Build history of the part. All positions in model axes, mm. A direction names the side the tool comes from. Round coordinates to 2 decimals unless told otherwise and drop trailing zeros. Write each loop counter-clockwise with the first axis right and the second up, starting at its lowest first coordinate (ties: lowest second). Pieces come first, ordered by that corner, then holes.
1) Saw through at A-A (z = 0). Write the cut outline in (x, y).
2) Wall check: probe 1 along X at (y, z) = (4.1, -137); probe 2 along Z at (x, y) = (6.5, 3.2); probe 3 along Z at (x, y) = (-5, 1.5). Give the ranges that are in metal, low to high.
3) Saw through at C-C (z = -32.5). Write the cut outline in (x, y).
4) Saw through at B-B (y = 4). State how many separate pieces and enclosed holes the cut face has, plus the area to 3 significant figures.
5) Pull direction Z, two halves, no side cores. Call faces 1 (the flat face through (11.13, 2.96, -147.46)), 2 (the flat face through (0, 3, -161)), 3 (the cylindrical face through (0.101, 2.958, 24.342)), 4 (the flat face through (14, 3, -18)): +Z half, -Z half, draft (parallel to the pull), parting line (faces both ways), or undercut.
6) Saw through at D-D (x = -15). Write the cut outline in (y, z).
7) Flat gauge pins, fed straight in: pin 1 (3 mm diameter, centred on x = 5, y = 2.5, fed in from -Z); pin 2 (3 mm diameter, centred on y = 1.5, z = -162, fed in from +X); pin 3 (1.8 mm diameter, centred on y = 3, z = -56, fed in from +X). Where does each tip first touch, or does it go through?
8) Which spindle directions (+Z, -Z, +X, -X, +Y, -Y) get a long thin tool onto all of the face, cutting with end or side? Do faces 5 (the cylindrical face through (0.33, 2.96, -122.61)), 6 (the flat face through (-12.5, 3, -118)), 7 (the flat face through (-7.6, 3, -56)), 8 (the flat face through (6, 3, -156.5)). Say none if no direction does.
Autodesk Inventor part; units mm, degrees
ref_plane "YZ Plane" through (0, 0, 0) normal (1, 0, 0) x (0, 1, 0)
ref_plane "XZ Plane" through (0, 0, 0) normal (0, 1, 0) x (-1, 0, 0)
ref_plane "XY Plane" through (0, 0, 0) normal (0, 0, 1) x (1, 0, 0)
sketch "Sketch1" plane through (0, 0, 0) normal (0, 1, 0) x (-1, 0, 0)
  line L0 (0, -158) -> (0, -165)
  arc A0 (1.5, -166.5) -> (0, -165) centre (0, -166.5) ccw
  line L1 (1.5, -166.5) -> (8.5, -166.5)
  arc A1 (8.5, -166.5) -> (10, -165) centre (8.5, -165) ccw
  line L2 (10, -165) -> (10, -156.5)
  line L3 (10, -156.5) -> (12.2297, -138.6622)
  arc A2 (12.2297, -138.6622) -> (12.5, -134.321) centre (-22.5, -134.321) ccw
  line L4 (12.5, -134.321) -> (12.5, -101.0909)
  arc A3 (12.5, -101.0909) -> (10.05, -91.4994) centre (-7.5, -101.0909) ccw
  arc A4 (7.6, -81.9079) -> (10.05, -91.4994) centre (27.6, -81.9079) ccw
  line L5 (7.6, -81.9079) -> (7.6, -29.8667)
  arc A5 (9.6, -23.8667) -> (7.6, -29.8667) centre (17.6, -29.8667) ccw
  line L6 (9.6, -23.8667) -> (18, -12.6667)
  arc A6 (18, -12.6667) -> (20, -6.6667) centre (10, -6.6667) ccw
  line L7 (20, -6.6667) -> (20, 5.4953)
  arc A7 (20, 5.4953) -> (16.6262, 12.9849) centre (10, 5.4953) ccw
  line L8 (16.6262, 12.9849) -> (6.6262, 21.8321)
  arc A8 (6.6262, 21.8321) -> (-6.6262, 21.8321) centre (0, 14.3426) ccw
  line L9 (-6.6262, 21.8321) -> (-16.6262, 12.9849)
  arc A9 (-16.6262, 12.9849) -> (-20, 5.4953) centre (-10, 5.4953) ccw
  line L10 (-20, 5.4953) -> (-20, -6.6667)
  arc A10 (-20, -6.6667) -> (-18, -12.6667) centre (-10, -6.6667) ccw
  line L11 (-18, -12.6667) -> (-9.6, -23.8667)
  arc A11 (-7.6, -29.8667) -> (-9.6, -23.8667) centre (-17.6, -29.8667) ccw
  line L12 (-7.6, -29.8667) -> (-7.6, -82.5915)
  arc A12 (-10.05, -92.183) -> (-7.6, -82.5915) centre (-27.6, -82.5915) ccw
  arc A13 (-10.05, -92.183) -> (-12.5, -101.7745) centre (7.5, -101.7745) ccw
  line L13 (-12.5, -101.7745) -> (-12.5, -134.321)
  arc A14 (-12.5, -134.321) -> (-12.2297, -138.6622) centre (22.5, -134.321) ccw
  line L14 (-12.2297, -138.6622) -> (-10, -156.5)
  line L15 (-10, -156.5) -> (-1.5, -156.5)
  arc A15 (0, -158) -> (-1.5, -156.5) centre (-1.5, -158) ccw
  arc A16 (-6.7529, 4.5608) -> (-4.5608, 6.7529) centre (-5.6569, 5.6569) ccw
  line L16 (-4.5608, 6.7529) -> (-5.6215, 7.8135)
  arc A17 (-5.6215, 7.8135) -> (-7.8135, 5.6215) centre (-6.7175, 6.7175) ccw
  line L17 (-7.8135, 5.6215) -> (-6.7529, 4.5608)
  line L18 (6.7529, -4.5608) -> (7.8135, -5.6215)
  arc A18 (5.6215, -7.8135) -> (7.8135, -5.6215) centre (6.7175, -6.7175) ccw
  line L19 (5.6215, -7.8135) -> (4.5608, -6.7529)
  arc A19 (6.7529, -4.5608) -> (4.5608, -6.7529) centre (5.6569, -5.6569) ccw
  line L20 (-7.8135, -5.6215) -> (-6.7529, -4.5608)
  arc A20 (-4.5608, -6.7529) -> (-6.7529, -4.5608) centre (-5.6569, -5.6569) ccw
  line L21 (-4.5608, -6.7529) -> (-5.6215, -7.8135)
  arc A21 (-7.8135, -5.6215) -> (-5.6215, -7.8135) centre (-6.7175, -6.7175) ccw
  line L22 (7.8135, 5.6215) -> (6.7529, 4.5608)
  arc A22 (4.5608, 6.7529) -> (6.7529, 4.5608) centre (5.6569, 5.6569) ccw
  line L23 (4.5608, 6.7529) -> (5.6215, 7.8135)
  arc A23 (7.8135, 5.6215) -> (5.6215, 7.8135) centre (6.7175, 6.7175) ccw
  circle A24 centre (0, 0) radius 3
  circle A25 centre (0, -124.0736) radius 1.5
  circle A26 centre (-6, -136.5) radius 1.5
  circle A27 centre (6, -136.5) radius 1.5
  circle A28 centre (0, -144.9332) radius 4
  point P0 (10, -165)
  point P1 (12.2297, -138.6622)
  point P2 (12.5, -101.0909)
  point P3 (10.05, -91.4994)
  point P4 (7.6, -81.9079)
  point P5 (7.6, -29.8667)
  point P6 (9.6, -23.8667)
  point P7 (20, -6.6667)
  point P8 (20, 5.4953)
  point P9 (16.6262, 12.9849)
  point P10 (6.6262, 21.8321)
  point P11 (-16.6262, 12.9849)
  point P12 (-20, 5.4953)
  point P13 (-9.6, -23.8667)
  point P14 (-10.05, -92.183)
  point P15 (-12.2297, -138.6622)
  point P16 (0, -158)
  point P17 (6.7529, -4.5608)
  point P18 (7.8135, -5.6215)
  point P19 (5.6215, -7.8135)
  point P20 (-7.8135, -5.6215)
  point P21 (-6.7529, -4.5608)
  point P22 (-4.5608, -6.7529)
  point P23 (-5.6215, -7.8135)
  point P24 (-5.6215, 7.8135)
  point P25 (-4.5608, 6.7529)
extrude "Extrusion1" add sketch "Sketch1" along normal blind 6
properties part number "TokerCNC froggy arm"
Evaluation:
1. outline: (-20, 0) - (-3, 0) - (-3, 6) - (-20, 6) - close; (3, 0) - (20, 0) - (20, 6) - (3, 6) - close
2. probe 1: x = -12.4 to -7.41, -4.59 to 4.59, 7.41 to 12.4
2. probe 2: z = -156.5 to -137.91, -135.09 to -8.25, -4.36 to 4.36, 8.25 to 21.94
2. probe 3: z = -166.5 to -137.62, -135.38 to -7.19, -4.25 to 4.25, 7.19 to 23
3. outline: (-7.6, 0) - (7.6, 0) - (7.6, 6) - (-7.6, 6) - close
4. separate pieces: 1
4. enclosed holes: 9
4. area: 4,100 mm2
5. face 1: -Z half
5. face 2: draft
5. face 3: +Z half
5. face 4: undercut
6. outline: (0, -16.67) - (6, -16.67) - (6, 14.42) - (0, 14.42) - close
7. pin 1: stops at z = -156.5
7. pin 2: stops at x = 0
7. pin 3: stops at x = 7.6
8. face 5: +Y, -Y
8. face 6: -Z, -X, +Y, -Y
8. face 7: -X, +Y, -Y
8. face 8: -Z, +X, +Y, -Y
